Check sheet for the modelled part. Datum: model origin and axes. Units: mm. A direction names the side the tool comes from. Round coordinates to 2 decimals unless told otherwise and drop trailing zeros. Write each loop counter-clockwise with the first axis right and the second up, starting at its lowest first coordinate (ties: lowest second). Pieces come first, ordered by that corner, then holes. Notation, with made-up numbers: (-23, 78) -> (20, 78) arc R35 ccw to (20, 112) -> close; hole circle Ø7 at (82.25, 79.25). An arc over 180 degrees is marked (long way). Write item = value, one per line.
from build123d import *

# Parameters (mm, degrees)
BOSS_EXTRUDE1_DEPTH = 200
CUT_EXTRUDE1_DEPTH  = 193
FILLET1_R           = 10
FILLET2_R           = 10
SKETCH5_W           = 221.977044751
SKETCH5_H           = 222.508090313
CUT_EXTRUDE2_DEPTH  = 2


with BuildPart() as part:
    # Sketch1 → Boss-Extrude1 (new body)
    with BuildSketch(Plane(origin=(0, 0, 0), x_dir=(1, 0, 0), z_dir=(0, 1, 0))):
        with BuildLine():
            Line((-80, 45), (80, 45))
            ThreePointArc((80, 45), (87.071067812, 42.071067812), (90, 35))
            Line((90, 35), (90, -35))
            Line((90, -35), (-90, -35))
            Line((-90, -35), (-90, 35))
            ThreePointArc((-90, 35), (-87.071067812, 42.071067812), (-80, 45))
        make_face()
    extrude(amount=-BOSS_EXTRUDE1_DEPTH)

    # Sketch2 → Cut-Extrude1 (cut)
    with BuildSketch(Plane(origin=(0, 0, 0), x_dir=(1, 0, 0), z_dir=(0, 1, 0))):
        with BuildLine():
            Line((85, -30), (85, 35))
            ThreePointArc((85, 35), (83.535533906, 38.535533906), (80, 40))
            Line((80, 40), (-80, 40))
            ThreePointArc((-80, 40), (-83.535533906, 38.535533906), (-85, 35))
            Line((-85, 35), (-85, -30))
            Line((-85, -30), (85, -30))
        make_face()
    extrude(amount=-CUT_EXTRUDE1_DEPTH, mode=Mode.SUBTRACT)

    # Fillet1
    fillet1_edges = [part.edges().sort_by_distance(p)[0] for p in [
        (0, -200, -45),
        (-87.071067812, -200, -42.071067812),
        (-90, -200, 0),
        (90, -200, 0),
        (87.071067812, -200, -42.071067812),
    ]]
    fillet(fillet1_edges, radius=FILLET1_R)

    # Fillet2
    # the kernel refuses this fillet: 10 mm, written as the material it takes off along each edge
    with BuildSketch(Plane(origin=(90, 0, -35), x_dir=(-1, 0, 0), z_dir=(0, 0, 1)), Plane(origin=(-90, 0, 60), x_dir=(1, 0, 0), z_dir=(0, 0, -1))) as fillet2_piece_1:
        with BuildLine():
            CenterArc((FILLET2_R, FILLET2_R), FILLET2_R, 180, 90)
            Line((0, FILLET2_R), (0, 0))
            Line((0, 0), (FILLET2_R, 0))
        make_face()
    extrude(amount=95, mode=Mode.SUBTRACT)
    with BuildSketch(Plane(origin=(-80, 0, -35), x_dir=(-1, 0, 0), z_dir=(0, 0, 1))) as fillet2_piece_2:
        with BuildLine():
            CenterArc((10 - FILLET2_R, FILLET2_R), FILLET2_R, 270, 90)
            Line((10 - FILLET2_R, 0), (10, 0))
            Line((10, 0), (10, FILLET2_R))
        make_face()
    revolve(axis=Axis((-80, 0, -35), (0, -1, 0)), revolution_arc=90, mode=Mode.SUBTRACT)
    with BuildSketch(Plane(origin=(-80, 0, -45), x_dir=(0, -1, 0), z_dir=(1, 0, 0))) as fillet2_piece_3:
        with BuildLine():
            CenterArc((FILLET2_R, -FILLET2_R), FILLET2_R, 90, 90)
            Line((0, -FILLET2_R), (0, 0))
            Line((0, 0), (FILLET2_R, 0))
        make_face()
    extrude(amount=160, mode=Mode.SUBTRACT)
    with BuildSketch(Plane(origin=(80, 0, -35), x_dir=(0, 0, -1), z_dir=(-1, 0, 0))) as fillet2_piece_4:
        with BuildLine():
            CenterArc((10 - FILLET2_R, FILLET2_R), FILLET2_R, 270, 90)
            Line((10, FILLET2_R), (10, 0))
            Line((10, 0), (10 - FILLET2_R, 0))
        make_face()
    revolve(axis=Axis((80, 0, -35), (0, -1, 0)), revolution_arc=90, mode=Mode.SUBTRACT)

    # Sketch5 → Cut-Extrude2 (cut)
    with BuildSketch(Plane.XY.offset(35)):
        with Locations((11.417479574, -99.417273917)):
            Rectangle(SKETCH5_W, SKETCH5_H)
    extrude(amount=-CUT_EXTRUDE2_DEPTH, mode=Mode.SUBTRACT)


solid = part.part
(1) Material ranges on L1, parallel to Z at x = 34, y = -86; L2, parallel to X at y = -96, z = -35; L3, parallel to Y at x = -76, z = 1, recorded low to high. Write a range as [from, to].
Worked answers:
L1 = [-45, -40], [30, 33]
L2 = [-90, -85], [85, 90]
L3 = [-200, -193]
(2) Go/stop test with a flat-tipped pin: P1, Ø4, axis at x = 33.5, z = -34.5, coming from the +Y side. Record where the tip stops, or that it passes through.
Worked answers:
P1 = -193
(3) Sectioned sample at B-B on z = -27. Enter the section's corners in (x, y).
Worked answers:
outline = (-90, -190) arc R10 ccw to (-80, -200) -> (80, -200) arc R10 ccw to (90, -190) -> (90, -10) arc R10 ccw to (85, -1.34) -> (85, -193) -> (-85, -193) -> (-85, -1.34) arc R10 ccw to (-90, -10) -> close
(4) Release check for a two-part mould opening along Z. For faces 3 (the flat face through (-1, -99, 33)), 4 (the flat face through (-90, -99, -1)), 5 (the cylindrical face through (1.12, -196.99, -42.15)), 6 (the flat face through (-1, -193, -5)) record: pulls with the +Z half, pulls with the -Z half, needs draft (parallel to the pull), parting line crosses it, or undercut.
Worked answers:
face_3 = pulls with the +Z half
face_4 = needs draft
face_5 = pulls with the -Z half
face_6 = undercut
(5) Sectioned sample at C-C on x = -70.5. Enter the section's corners in (y, z).
Worked answers:
outline = (-200, -35) arc R10 ccw to (-190, -45) -> (-10, -45) arc R10 ccw to (-1.34, -40) -> (-193, -40) -> (-193, 30) -> (0, 30) -> (0, 33) -> (-200, 33) -> close
(6) Access from +Z, -Z, +X, -X, +Y, -Y to the whole of each face (thin tool, end or side, straight path). Record for faces 1 (the cylindrical face through (86.99, -98.74, -42.15)), 2 (the cylindrical face through (84, -96, -38)).
Worked answers:
face_1 = -Z, +X, +Y, -Y
face_2 = +Y
(7) Sectioned sample at A-A on y = -162. Enter the section's corners in (x, z).
Worked answers:
outline = (-90, -35) arc R10 ccw to (-80, -45) -> (80, -45) arc R10 ccw to (90, -35) -> (90, 33) -> (-90, 33) -> close; hole (-85, -35) arc R5 ccw to (-80, -40) -> (80, -40) arc R5 ccw to (85, -35) -> (85, 30) -> (-85, 30) -> close
